For this review, take the finished solid that the model builds, in its own axes (mm). A direction names the side the tool comes from. Give positions to 0.01 mm unless a question says otherwise; leave off trailing zeros. Write each loop counter-clockwise with the first axis right and the second up, starting at its lowest first coordinate (ties: lowest second). Pieces come first, ordered by that corner, then holes.
Q1. Machinability: for faces 1 (the cylindrical face through (5.137, -1.138, 5.077)), 2 (the cylindrical face through (-0.33, -5.12, 2.52)), which of the approach directions +Z, -Z, +X, -X, +Y, -Y give a long, thin tool a straight path to every point of the face, cutting with its end or side? Answer none if there is none.
Q2. We need section C-C (y = -3). Write out the cut boundary in (x, z), then the cut area to 3 significant figures.
Q3. For line 1 (Y direction, x = 1, z = -3.5); line 2 (X direction, y = -4.25, z = 0.25); line 3 (X direction, y = -1.75, z = 2), list the stretches that pass through material, from the lowest coordinate up.
Q4. We need section B-B (z = 0). Write out the cut boundary in (x, y).
Q5. We need section A-A (x = 0). Write out the cut boundary in (y, z), then the cut area to 3 significant figures.
Q6. Insertion check: P1, Ø1, axis at y = -5.5, z = 4.5, coming from the -X side; P2, Ø3, axis at x = -3.5, y = -4, coming from the +Z side; P3, Ø2, axis at x = -2, y = -3.5, coming from the +Z side; P4, Ø5, axis at x = -5, z = -3, coming from the -Y side. Each pin has a flat end and moves straight along its axis. Give the tip position at first contact, or say it passes through.
Q7. We need section D-D (x = -3). Write out the cut boundary in (y, z), then the cut area to 3 significant figures.
```python
from build123d import *

# Parameters (mm, degrees)
F1_DEPTH = 1.524
F2_R     = 0.762
F3_R     = 2.54
F4_DEPTH = 7.874
F5_SIZE2 = 1.016
F5_SIZE  = 0.5865878735


with BuildPart() as f1:
    # F0 (on Front) → F1 (new body)
    with BuildSketch(Plane.XZ):
        with BuildLine():
            ThreePointArc((6.223, 2.413), (5.1070768363, 5.1070768363), (2.413, 6.223))
            Line((2.413, 6.223), (-5.461, 6.223))
            ThreePointArc((-5.461, 6.223), (-5.9998153673, 5.9998153673), (-6.223, 5.461))
            Line((-6.223, 5.461), (-6.223, -5.461))
            ThreePointArc((-6.223, -5.461), (-5.9998153673, -5.9998153673), (-5.461, -6.223))
            Line((-5.461, -6.223), (2.413, -6.223))
            ThreePointArc((2.413, -6.223), (5.1070768363, -5.1070768363), (6.223, -2.413))
            Line((6.223, -2.413), (6.223, 2.413))
        make_face()
    extrude(amount=F1_DEPTH)

    # F2
    f2_edges = [f1.edges().sort_by_distance(p)[0] for p in [
        (-1.524, 0, -6.223),
    ]]
    fillet(f2_edges, radius=F2_R)

    # F3 (on face) → F4 (join)
    with BuildSketch(Plane.XZ.offset(1.524)):
        Circle(F3_R)
    extrude(amount=F4_DEPTH)

    # F5
    f5_edges = [f1.edges().sort_by_distance(p)[0] for p in [
        (-2.54, -9.398, 0),
    ]]
    f5_side = f1.faces().sort_by_distance((-2.54, -5.461, 0))[0]
    chamfer(f5_edges, length=F5_SIZE, length2=F5_SIZE2, reference=f5_side)


solid = f1.part
```
Computed:
1. face 1: +Z, +X, +Y, -Y
1. face 2: -Y
2. outline: circle Ø5.08 at (0, 0)
2. area: 20.3 mm2
3. line 1: y = -1.52 to 0
3. line 2: x = -2.53 to 2.53
3. line 3: x = -1.57 to 1.57
4. outline: (-6.22, -1.52) - (-2.54, -1.52) - (-2.54, -8.81) - (-1.52, -9.4) - (1.52, -9.4) - (2.54, -8.81) - (2.54, -1.52) - (6.22, -1.52) - (6.22, -0.76) arc R0.76 ccw to (5.46, 0) - (-5.46, 0) arc R0.76 ccw to (-6.22, -0.76) - close
5. outline: (-9.4, -1.52) - (-8.81, -2.54) - (-1.52, -2.54) - (-1.52, -6.22) - (-0.76, -6.22) arc R0.76 ccw to (0, -5.46) - (0, 5.46) arc R0.76 ccw to (-0.76, 6.22) - (-1.52, 6.22) - (-1.52, 2.54) - (-8.81, 2.54) - (-9.4, 1.52) - close
5. area: 58.1 mm2
6. P1: passes through
6. P2: stops at z = 1.57
6. P3: stops at z = 2.33
6. P4: stops at y = -1.52
7. outline: (-1.52, -6.22) - (-0.76, -6.22) arc R0.76 ccw to (0, -5.46) - (0, 5.46) arc R0.76 ccw to (-0.76, 6.22) - (-1.52, 6.22) - close
7. area: 18.7 mm2
